For this review, take the finished solid that the model builds, in its own axes (mm). Face numbers are marked on the shaded views. Round coordinates to 2 decimals unless told otherwise and drop trailing zeros. Loops run counter-clockwise (first coordinate to the right, second up) from the corner with the lowest first, then second, coordinate; pieces in that order, holes last. Notation, with made-up numbers: (26, 89) -> (69, 89) arc R28 ccw to (69, 116) -> close; hole circle Ø5 at (-20.75, -24). An arc over 180 degrees is marked (long way). Write each question's results on one line, items separated by ' | '.
```python
from build123d import *

# Parameters (mm, degrees)
SKETCH1_W           = 266.7
SKETCH1_H           = 101.6
SKETCH1_R           = 9.8425
SKETCH1_R_2         = 3.429
BOSS_EXTRUDE1_DEPTH = 19.05
FILLET1_R           = 10
SKETCH2_R           = 7.5
CUT_EXTRUDE1_DEPTH  = 5.842


with BuildPart() as part:
    # Sketch1 → Boss-Extrude1 (new body)
    with BuildSketch(Plane(origin=(0, 0, 0), x_dir=(1, 0, 0), z_dir=(0, 1, 0))):
        with Locations((133.35, 50.8)):
            Rectangle(SKETCH1_W, SKETCH1_H)
        with Locations(Location((31.75, 25.4, 0), (0, 0, 270))):  # turned: the seam where the file's is
            Circle(SKETCH1_R, mode=Mode.SUBTRACT)
        with Locations(Location((82.55, 25.4, 0), (0, 0, 270))):  # turned: the seam where the file's is
            Circle(SKETCH1_R, mode=Mode.SUBTRACT)
        with Locations(Location((133.35, 25.4, 0), (0, 0, 270))):  # turned: the seam where the file's is
            Circle(SKETCH1_R, mode=Mode.SUBTRACT)
        with Locations(Location((184.15, 25.4, 0), (0, 0, 270))):  # turned: the seam where the file's is
            Circle(SKETCH1_R, mode=Mode.SUBTRACT)
        with Locations(Location((234.95, 25.4, 0), (0, 0, 270))):  # turned: the seam where the file's is
            Circle(SKETCH1_R, mode=Mode.SUBTRACT)
        with Locations(Location((82.55, 76.2, 0), (0, 0, 270))):  # turned: the seam where the file's is
            Circle(SKETCH1_R, mode=Mode.SUBTRACT)
        with Locations(Location((133.35, 76.2, 0), (0, 0, 270))):  # turned: the seam where the file's is
            Circle(SKETCH1_R, mode=Mode.SUBTRACT)
        with Locations(Location((184.15, 76.2, 0), (0, 0, 270))):  # turned: the seam where the file's is
            Circle(SKETCH1_R, mode=Mode.SUBTRACT)
        with Locations(Location((234.95, 76.2, 0), (0, 0, 270))):  # turned: the seam where the file's is
            Circle(SKETCH1_R, mode=Mode.SUBTRACT)
        with Locations(Location((31.75, 76.2, 0), (0, 0, 270))):  # turned: the seam where the file's is
            Circle(SKETCH1_R, mode=Mode.SUBTRACT)
        with Locations(Location((9.525, 92.075, 0), (0, 0, 270))):  # turned: the seam where the file's is
            Circle(SKETCH1_R_2, mode=Mode.SUBTRACT)
        with Locations(Location((257.175, 92.075, 0), (0, 0, 90))):  # turned: the seam where the file's is
            Circle(SKETCH1_R_2, mode=Mode.SUBTRACT)
        with Locations(Location((9.525, 9.525, 0), (0, 0, 90))):  # turned: the seam where the file's is
            Circle(SKETCH1_R_2, mode=Mode.SUBTRACT)
        with Locations(Location((257.175, 9.525, 0), (0, 0, 270))):  # turned: the seam where the file's is
            Circle(SKETCH1_R_2, mode=Mode.SUBTRACT)
    extrude(amount=BOSS_EXTRUDE1_DEPTH)

    # Fillet1
    fillet1_edges = [part.edges().sort_by_distance(p)[0] for p in [
        (0, 9.525, -101.6),
        (266.7, 9.525, -101.6),
        (266.7, 9.525, 0),
        (0, 9.525, 0),
    ]]
    fillet(fillet1_edges, radius=FILLET1_R)

    # Sketch2 → Cut-Extrude1 (cut)
    with BuildSketch(Plane(origin=(0, 19.05, 0), x_dir=(1, 0, 0), z_dir=(0, 1, 0))):
        with Locations(Location((9.525, 92.075, 0), (0, 0, 270))):  # turned: the seam where the file's is
            Circle(SKETCH2_R)
        with Locations(Location((257.175, 92.075, 0), (0, 0, 270))):  # turned: the seam where the file's is
            Circle(SKETCH2_R)
        with Locations(Location((257.175, 9.525, 0), (0, 0, 270))):  # turned: the seam where the file's is
            Circle(SKETCH2_R)
        with Locations(Location((9.525, 9.525, 0), (0, 0, 270))):  # turned: the seam where the file's is
            Circle(SKETCH2_R)
    extrude(amount=-CUT_EXTRUDE1_DEPTH, mode=Mode.SUBTRACT)


solid = part.part
```
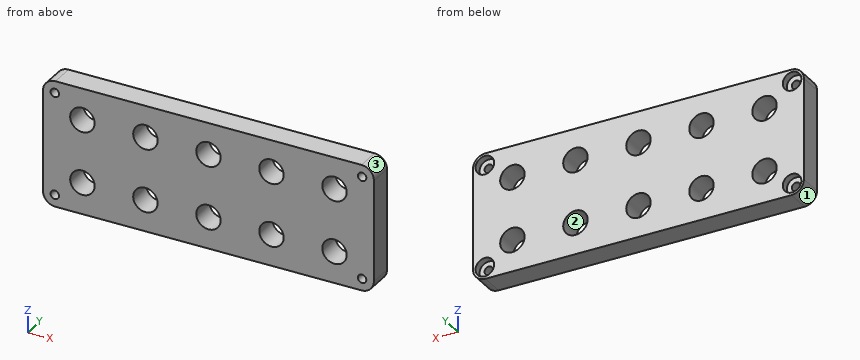
1. Draft analysis for pull direction Z (two halves, no side actions). For the marked faces 1, 2 and 3, state which applies: released by +Z, released by -Z, zero draft, split by the parting line, or undercut.
Values found:
face 1: released by -Z | face 2: undercut | face 3: released by +Z
2. To check wall thickness, follow probe 1 along Z at (x, y) = (83, 12); probe 2 along Z at (x, y) = (236.5, 12.5); probe 3 along X at (y, z) = (4.5, -93). State the ranges of each line that lie inside material, in increasing order.
Values found:
probe 1: z = -101.6 to -86.03, -66.37 to -35.23, -15.57 to 0 | probe 2: z = -101.6 to -85.92, -66.48 to -35.12, -15.68 to 0 | probe 3: x = 0.1 to 6.22, 12.83 to 253.87, 260.48 to 266.6
3. Consider section A-A (z = -25.4). State the section outline as (x, y) points, plus the area to 3 significant figures.
Values found:
outline: (0, 0) -> (21.91, 0) -> (21.91, 19.05) -> (0, 19.05) -> close; (41.59, 0) -> (72.71, 0) -> (72.71, 19.05) -> (41.59, 19.05) -> close; (92.39, 0) -> (123.51, 0) -> (123.51, 19.05) -> (92.39, 19.05) -> close; (143.19, 0) -> (174.31, 0) -> (174.31, 19.05) -> (143.19, 19.05) -> close; (193.99, 0) -> (225.11, 0) -> (225.11, 19.05) -> (193.99, 19.05) -> close; (244.79, 0) -> (266.7, 0) -> (266.7, 19.05) -> (244.79, 19.05) -> close | area: 3,210 mm2
4. Consider section C-C (y = 10.5). Give the number of separate pieces and of enclosed holes in the cut face, plus the area to 3 significant figures.
Values found:
separate pieces: 1 | enclosed holes: 14 | area: 23,800 mm2
5. Consider section D-D (x = 136.5). State the section outline as (y, z) points, plus the area to 3 significant figures.
Values found:
outline: (0, -101.6) -> (19.05, -101.6) -> (19.05, -85.52) -> (0, -85.52) -> close; (0, -66.88) -> (19.05, -66.88) -> (19.05, -34.72) -> (0, -34.72) -> close; (0, -16.08) -> (19.05, -16.08) -> (19.05, 0) -> (0, 0) -> close | area: 1,220 mm2
6. Consider section B-B (x = 31.75). State the section outline as (y, z) points.
Values found:
outline: (0, -101.6) -> (19.05, -101.6) -> (19.05, -86.04) -> (0, -86.04) -> close; (0, -66.36) -> (19.05, -66.36) -> (19.05, -35.24) -> (0, -35.24) -> close; (0, -15.56) -> (19.05, -15.56) -> (19.05, 0) -> (0, 0) -> close
7. For pin 1 (22.5 mm diameter, centred on x = 82.55, z = -76.2, fed in from -Y); pin 2 (11 mm diameter, centred on x = 9.525, z = -9.525, fed in from +Y), all flat-tipped, find the tip position at first contact; note any pin that passes through.
Values found:
pin 1: stops at y = 0 | pin 2: stops at y = 13.21
